from build123d import *

# Parameters (mm, degrees)
BOSS_EXTRUDE1_DEPTH = 20.32
SKETCH2_W           = 120.284747719
SKETCH2_H           = 10.16
SKETCH2_W_2         = 118.872828106
SKETCH2_W_3         = 10.166490401
SKETCH2_H_2         = 89.916
SKETCH2_W_4         = 102.891608588
SKETCH2_W_5         = 94.453494602
SKETCH2_W_6         = 3.175
SKETCH2_W_7         = 561.9496
CUT_EXTRUDE1_DEPTH  = 137.414
SKETCH3_W           = 337.058
SKETCH3_H           = 124.46
CUT_EXTRUDE2_DEPTH  = 137.414
SKETCH4_W           = 10.16
SKETCH4_H           = 63.685061479
SKETCH4_H_2         = 63.685061478
CUT_EXTRUDE3_DEPTH  = 20.32
SKETCH10_R          = 3.175
CUT_EXTRUDE5_DEPTH  = 20.32
SKETCH12_R          = 4.7625
CUT_EXTRUDE6_DEPTH  = 917.604828076
SKETCH14_R          = 3.175
CUT_EXTRUDE7_DEPTH  = 917.604828076
SKETCH15_R          = 4.7625
SKETCH15_R_2        = 3.175
CUT_EXTRUDE8_DEPTH  = 917.604828076
SKETCH16_W          = 585.62283163
SKETCH16_H          = 602.215256286
SKETCH16_W_2        = 414.697903798
SKETCH16_H_2        = 659.676019196
CUT_EXTRUDE9_DEPTH  = 25.4


with BuildPart() as part:
    # Sketch1 → Boss-Extrude1 (new body)
    with BuildSketch(Plane.XY):
        Polygon((94.041322477, 150.485716341), (-175.036761108, 150.485716341), (-142.097719316, 314.8709952), (61.102280684, 314.8709952), align=None)
        with BuildLine():
            Line((-606.997271248, -319.414283659), (526.001832617, -319.414283659))
            add(Edge.make_bspline(
                [(583.362059287, -282.457957765), (581.029219579, -287.649310181), (577.879080401, -292.734699958), (570.038270446, -301.965622016), (565.348976837, -306.100497209), (554.949172694, -312.800933616), (549.248266441, -315.360306939), (537.611112797, -318.678742027), (531.685117348, -319.440968422), (526.001832617, -319.414283659)],
                knots=[0, 0, 0, 0, 0.25, 0.25, 0.5, 0.5, 0.75, 0.75, 1, 1, 1, 1], degree=3))
            Line((583.362059287, -282.457957765), (777.91409763, 150.485716341))
            Line((777.91409763, 150.485716341), (-858.909536262, 150.485716341))
            Line((-858.909536262, 150.485716341), (-664.600308277, -281.91762311))
            add(Edge.make_bspline(
                [(-664.600308277, -281.91762311), (-662.275037436, -287.157802838), (-659.126015856, -292.295113907), (-651.27178065, -301.630322109), (-646.567903812, -305.817478055), (-636.124076479, -312.615880857), (-630.393770919, -315.220849348), (-618.687590773, -318.618481158), (-612.722057732, -319.414283659), (-606.997271248, -319.414283659)],
                knots=[0, 0, 0, 0, 0.25, 0.25, 0.5, 0.5, 0.75, 0.75, 1, 1, 1, 1], degree=3))
        make_face()
    extrude(amount=BOSS_EXTRUDE1_DEPTH)

    # Sketch2 → Cut-Extrude1 (cut)
    with BuildSketch(Plane(origin=(0, 0, 0), x_dir=(-1, 0, 0), z_dir=(0, 0, -1))):
        with Locations((-547.078117621, 145.405716341)):
            Rectangle(SKETCH2_W, SKETCH2_H)
        with Locations((-307.214581989, 145.405716341)):
            Rectangle(SKETCH2_W_2, SKETCH2_H)
        with Locations((-271.919035422, 5.451716341)):
            Rectangle(SKETCH2_W_3, SKETCH2_H_2)
        with Locations((-271.919035422, -174.380283659)):
            Rectangle(SKETCH2_W_3, SKETCH2_H_2)
        with Locations((352.914474055, -174.380283659)):
            Rectangle(SKETCH2_W_3, SKETCH2_H_2)
        with Locations((352.914474055, 5.451716341)):
            Rectangle(SKETCH2_W_3, SKETCH2_H_2)
        with Locations((380.219410862, 145.405716341)):
            Rectangle(SKETCH2_W_4, SKETCH2_H)
        with Locations((586.002628038, 145.405716341)):
            Rectangle(SKETCH2_W_4, SKETCH2_H)
        with Locations((-382.157322587, -314.334283659)):
            Rectangle(SKETCH2_W_5, SKETCH2_H)
        with Locations((463.152761219, -314.334283659)):
            Rectangle(SKETCH2_W_5, SKETCH2_H)
        with Locations((-278.589780623, -174.380283659)):
            Rectangle(SKETCH2_W_6, SKETCH2_H_2)
        with Locations((-265.248290222, -174.380283659)):
            Rectangle(SKETCH2_W_6, SKETCH2_H_2)
        with Locations((-278.589780623, 5.451716341)):
            Rectangle(SKETCH2_W_6, SKETCH2_H_2)
        with Locations((-265.248290222, 5.451716341)):
            Rectangle(SKETCH2_W_6, SKETCH2_H_2)
        with Locations((346.243728854, 5.451716341)):
            Rectangle(SKETCH2_W_6, SKETCH2_H_2)
        with Locations((359.585219255, 5.451716341)):
            Rectangle(SKETCH2_W_6, SKETCH2_H_2)
        with Locations((346.243728854, -174.380283659)):
            Rectangle(SKETCH2_W_6, SKETCH2_H_2)
        with Locations((359.585219255, -174.380283659)):
            Rectangle(SKETCH2_W_6, SKETCH2_H_2)
        with Locations((40.497719316, -314.334283659)):
            Rectangle(SKETCH2_W_7, SKETCH2_H)
    extrude(amount=-CUT_EXTRUDE1_DEPTH, mode=Mode.SUBTRACT)

    # Sketch3 → Cut-Extrude2 (cut)
    with BuildSketch(Plane.XY.offset(20.32)):
        with Locations((-40.497719316, -257.184283659)):
            Rectangle(SKETCH3_W, SKETCH3_H)
    extrude(amount=-CUT_EXTRUDE2_DEPTH, mode=Mode.SUBTRACT)

    # Sketch4 → Cut-Extrude3 (cut)
    with BuildSketch(Plane(origin=(0, 0, 0), x_dir=(-1, 0, 0), z_dir=(0, 0, -1))):
        Polygon((-160.162280684, -245.551796758), (-160.162280684, -309.254283659), (-128.031280684, -309.254283659), (-128.031280684, -194.954283659), (-150.002280684, -194.954283659), (-150.002280684, -245.551796758), align=None)
        Polygon((241.157719316, -309.254283659), (241.157719316, -245.551796758), (230.997719316, -245.551796758), (230.997719316, -194.954283659), (209.026719316, -194.954283659), (209.026719316, -309.254283659), align=None)
        with Locations((-155.082280684, -150.02420454)):
            Rectangle(SKETCH4_W, SKETCH4_H)
        with Locations((-155.082280684, -22.654081584)):
            Rectangle(SKETCH4_W, SKETCH4_H)
        with Locations((-155.082280684, 104.698615951)):
            Rectangle(SKETCH4_W, SKETCH4_H_2)
        with Locations((236.077719316, -150.02420454)):
            Rectangle(SKETCH4_W, SKETCH4_H)
        with Locations((236.077719316, -22.654081584)):
            Rectangle(SKETCH4_W, SKETCH4_H)
        with Locations((236.077719316, 104.698615951)):
            Rectangle(SKETCH4_W, SKETCH4_H_2)
    extrude(amount=-CUT_EXTRUDE3_DEPTH, mode=Mode.SUBTRACT)

    # Sketch10 → Cut-Extrude5 (cut)
    with BuildSketch(Plane.XY):
        with Locations((372.252552874, 80.840970313)):
            Circle(SKETCH10_R)
        with Locations((296.052552874, 80.840970313)):
            Circle(SKETCH10_R)
        with Locations((296.052552874, -8.059029687)):
            Circle(SKETCH10_R)
        with Locations((338.076100273, -8.059019539)):
            Circle(SKETCH10_R)
        with Locations((296.052552874, -96.959029687)):
            Circle(SKETCH10_R)
        with Locations((327.929280684, -242.858683659)):
            Circle(SKETCH10_R)
        with Locations((327.929280684, -268.258683659)):
            Circle(SKETCH10_R)
        with Locations((429.529280684, -268.258683659)):
            Circle(SKETCH10_R)
        with Locations((429.529280684, -242.858683659)):
            Circle(SKETCH10_R)
        with Locations(Location((-510.524719316, -242.858683659, 0), (0, 0, 180))):
            Circle(SKETCH10_R)
        with Locations(Location((-510.524719316, -268.258683659, 0), (0, 0, 180))):
            Circle(SKETCH10_R)
        with Locations(Location((-408.924719316, -268.258683659, 0), (0, 0, 180))):
            Circle(SKETCH10_R)
        with Locations(Location((-408.924719316, -242.858683659, 0), (0, 0, 180))):
            Circle(SKETCH10_R)
        with Locations(Location((-377.047991505, -96.959029687, 0), (0, 0, 180))):
            Circle(SKETCH10_R)
        with Locations(Location((-419.071538905, -8.059019539, 0), (0, 0, 180))):
            Circle(SKETCH10_R)
        with Locations(Location((-377.047991505, -8.059029687, 0), (0, 0, 180))):
            Circle(SKETCH10_R)
        with Locations(Location((-377.047991505, 80.840970313, 0), (0, 0, 180))):
            Circle(SKETCH10_R)
        with Locations(Location((-453.247991505, 80.840970313, 0), (0, 0, 180))):
            Circle(SKETCH10_R)
    extrude(amount=CUT_EXTRUDE5_DEPTH, mode=Mode.SUBTRACT)

    # Sketch12 → Cut-Extrude6 (cut, through all)
    with BuildSketch(Plane(origin=(0, 0, 0), x_dir=(-1, 0, 0), z_dir=(0, 0, -1))):
        with Locations((-41.226780684, 125.085716341)):
            Circle(SKETCH12_R)
        with Locations((-41.226780684, 23.485716341)):
            Circle(SKETCH12_R)
        with Locations((-131.777780684, 23.485716341)):
            Circle(SKETCH12_R)
        with Locations((-131.777780684, 125.085716341)):
            Circle(SKETCH12_R)
        with Locations((212.773219316, 23.485716341)):
            Circle(SKETCH12_R)
        with Locations((212.773219316, 125.085716341)):
            Circle(SKETCH12_R)
        with Locations((122.222219316, 125.085716341)):
            Circle(SKETCH12_R)
        with Locations((122.222219316, 23.485716341)):
            Circle(SKETCH12_R)
    extrude(amount=-CUT_EXTRUDE6_DEPTH, mode=Mode.SUBTRACT)

    # Sketch14 → Cut-Extrude7 (cut, through all)
    with BuildSketch(Plane.XY.offset(20.32)):
        with Locations((435.255534848, 113.379343598)):
            Circle(SKETCH14_R)
        with Locations((485.903167936, 96.510716341)):
            Circle(SKETCH14_R)
        with Locations((485.903167936, 130.247970855)):
            Circle(SKETCH14_R)
    extrude(amount=-CUT_EXTRUDE7_DEPTH, mode=Mode.SUBTRACT)

    # Sketch15 → Cut-Extrude8 (cut, through all)
    with BuildSketch(Plane(origin=(0, 0, 0), x_dir=(-1, 0, 0), z_dir=(0, 0, -1))):
        with Locations((-54.752280684, -87.004283659)):
            Circle(SKETCH15_R)
        with Locations((135.747719316, -87.004283659)):
            Circle(SKETCH15_R)
        with Locations((40.497719316, -80.654283659)):
            Circle(SKETCH15_R_2)
    extrude(amount=-CUT_EXTRUDE8_DEPTH, mode=Mode.SUBTRACT)

    # Sketch16 → Cut-Extrude9 (cut)
    with BuildSketch(Plane(origin=(0, 0, 0), x_dir=(-1, 0, 0), z_dir=(0, 0, -1))):
        with Locations((810.161921947, -112.521911802)):
            Rectangle(SKETCH16_W, SKETCH16_H)
        with Locations((-643.704019399, -141.252293257)):
            Rectangle(SKETCH16_W_2, SKETCH16_H_2)
    extrude(amount=-CUT_EXTRUDE9_DEPTH, mode=Mode.SUBTRACT)


solid = part.part
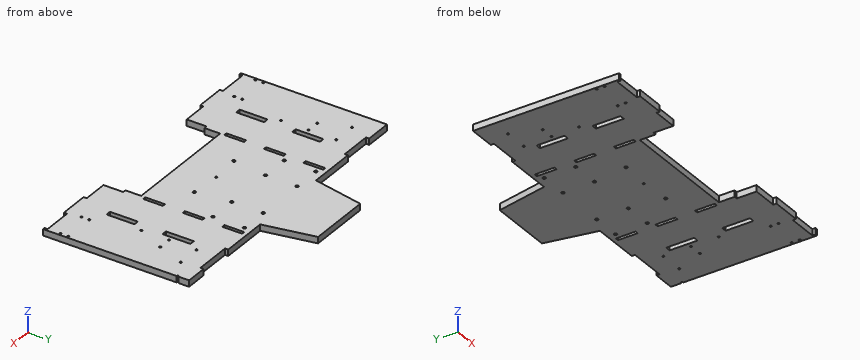
Work out the finished part from the listing and answer in its coordinate system (mm). Round coordinates to 2 decimals unless told otherwise and drop trailing zeros. Write each loop counter-clockwise with the first axis right and the second up, starting at its lowest first coordinate (ties: lowest second). Pieces come first, ordered by that corner, then holes.
1) A cutting plane is placed at A-A (x = -20.5). Give the vertices of the cut face in (y, z).
2) Given pin 1 Ø6 at (x, z) = (-23.5, 16.5) entering from -Y; pin 2 Ø1.5 at (x, z) = (-233, 3.5) entering from +Y; pin 3 Ø10 at (x, z) = (-276.5, 13.5) entering from -Y, each flat-ended and moving along its own axis, determine where each tip first touches the part or whether it passes through.
3) A cutting plane is placed at B-B (y = 175). Give the vertices of the cut face in (x, z), plus the area to 3 significant figures.
4) A cutting plane is placed at C-C (z = 10.5). Give the number of separate pieces and of enclosed holes in the cut face, plus the area to 3 significant figures.
5) Straight lines are drawn through the part: line 1 (Y direction, x = -350, z = 18); line 2 (X direction, y = -170, z = 13); line 3 (X direction, y = 149, z = 4.25). For each, find the intervals that lie inside material, in ascending order.
Completed:
1. outline: (-194.95, 0) - (314.87, 0) - (314.87, 20.32) - (-194.95, 20.32) - close
2. pin 1: stops at y = -194.95
2. pin 2: stops at y = 150.49
2. pin 3: stops at y = -309.25
3. outline: (-170.12, 0) - (89.13, 0) - (89.13, 20.32) - (-170.12, 20.32) - close
3. area: 5,270 mm2
4. separate pieces: 1
4. enclosed holes: 39
4. area: 421,000 mm2
5. line 1: y = -319.41 to -219.34, -129.42 to -39.51, 50.41 to 140.33
5. line 2: x = -517.35 to -361.17, -344.66 to -241.16, -231 to 150, 160.16 to 263.66, 280.18 to 436.36
5. line 3: x = -517.35 to -431.67, -328.77 to 247.78, 366.65 to 436.36
